Input: part model. Units: mm. Frame: model coordinates. Face numbers are marked on the shaded views. A direction names the side the tool comes from. Give positions to 0.01 mm unless a question says otherwise; leave off trailing zeros. Loops run counter-clockwise (first coordinate to the right, second up) from the corner with the lowest first, then second, coordinate; pieces in that order, holes last.
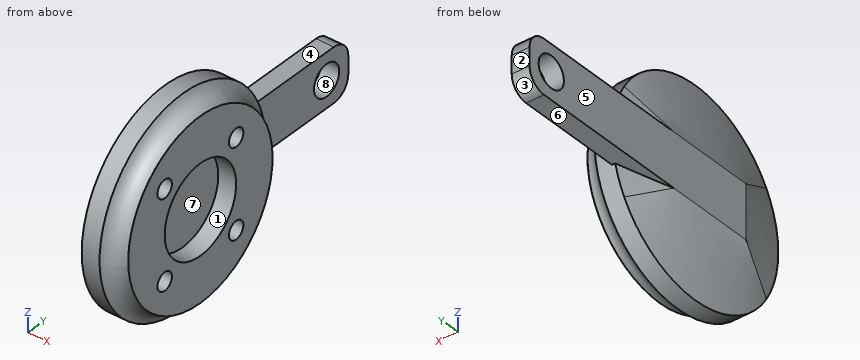
from build123d import *

# Parameters (mm, degrees)
SKETCH1_R           = 11.5
SKETCH1_R_2         = 10.5
BOSS_EXTRUDE1_DEPTH = 2
SKETCH1_2_R         = 10.5
BOSS_EXTRUDE2_DEPTH = 2
SKETCH3_R           = 9.5
CUT_EXTRUDE2_DEPTH  = 1.5
SKETCH6_W           = 30
SKETCH6_H           = 6
SKETCH6_R           = 1.75
BOSS_EXTRUDE3_DEPTH = 2
SKETCH7_R           = 10
SKETCH7_R_2         = 1
SKETCH7_R_3         = 4.95
BOSS_EXTRUDE4_DEPTH = 2
FILLET1_R           = 2
FILLET2_R           = 2


with BuildPart() as part:
    # Sketch1 → Boss-Extrude1 (new body)
    with BuildSketch(Plane.YZ):
        with Locations(Location((0, 0, 0), (0, 0, 270))):
            Circle(SKETCH1_R)
        with Locations(Location((0, 0, 0), (0, 0, 270))):
            Circle(SKETCH1_R_2, mode=Mode.SUBTRACT)
    extrude(amount=BOSS_EXTRUDE1_DEPTH)

    # Sketch1<2> → Boss-Extrude2 (add)
    with BuildSketch(Plane.YZ):
        Circle(SKETCH1_2_R)
    extrude(amount=BOSS_EXTRUDE2_DEPTH)

    # Sketch3 → Cut-Extrude2 (cut)
    with BuildSketch(Plane(origin=(0, 0, 0), x_dir=(0, -1, 0), z_dir=(-1, 0, 0))):
        with Locations(Location((0, 0, 0), (0, 0, 90))):
            Circle(SKETCH3_R)
    extrude(amount=-CUT_EXTRUDE2_DEPTH, mode=Mode.SUBTRACT)

    # Sketch4 for Loft1 → Loft1 section 0
    with BuildSketch(Plane(origin=(0, 0, 0), x_dir=(0, -1, 0), z_dir=(-1, 0, 0))):
        with BuildLine():
            # circular arc as an exact rational Bezier (weights 1, cos(half-angle), 1)
            Bezier((9.861168646, -5.916701187), (13.411189358, 0), (9.861168646, 5.916701187), weights=[1, 0.857492926, 1])
            Bezier((9.861168646, 5.916701187), (0, 22.351982265), (-9.861168646, 5.916701187), weights=[1, 0.514495755, 1])
            Bezier((-9.861168646, 5.916701187), (-13.411189358, 0), (-9.861168646, -5.916701187), weights=[1, 0.857492926, 1])
            Bezier((-9.861168646, -5.916701187), (0, -22.351982265), (9.861168646, -5.916701187), weights=[1, 0.514495755, 1])
        make_face()
    # Sketch2 → Loft1 section 1
    with BuildSketch(Plane.ZY.offset(1.64)):
        with BuildLine():
            Line((-3, -5), (3, -5))
            Line((3, -5), (3, 5))
            Line((3, 5), (-3, 5))
            Line((-3, 5), (-3, -5))
        make_face()
    loft()

    # Sketch6 → Boss-Extrude3 (add)
    with BuildSketch(Plane(origin=(-1.64, 0, 0), x_dir=(0, -1, 0), z_dir=(-1, 0, 0))):
        with Locations((-10, 0)):
            Rectangle(SKETCH6_W, SKETCH6_H)
        with Locations(Location((-22, 0, 0), (0, 0, 90))):
            Circle(SKETCH6_R, mode=Mode.SUBTRACT)
    extrude(amount=-BOSS_EXTRUDE3_DEPTH)

    # Sketch7 → Boss-Extrude4 (add)
    with BuildSketch(Plane.YZ.offset(2)):
        with Locations(Location((0, 0, 0), (0, 0, 270))):
            Circle(SKETCH7_R)
        with Locations(Location((-4.95, 4.95, 0), (0, 0, 270))):
            Circle(SKETCH7_R_2, mode=Mode.SUBTRACT)
        with Locations(Location((4.95, 4.95, 0), (0, 0, 270))):
            Circle(SKETCH7_R_2, mode=Mode.SUBTRACT)
        with Locations(Location((4.95, -4.95, 0), (0, 0, 270))):
            Circle(SKETCH7_R_2, mode=Mode.SUBTRACT)
        with Locations(Location((-4.95, -4.95, 0), (0, 0, 270))):
            Circle(SKETCH7_R_2, mode=Mode.SUBTRACT)
        with Locations(Location((0, 0, 0), (0, 0, 270))):
            Circle(SKETCH7_R_3, mode=Mode.SUBTRACT)
    extrude(amount=BOSS_EXTRUDE4_DEPTH)

    # Fillet1
    # the kernel refuses this fillet: 2 mm, written as the material it adds along each edge
    with BuildSketch(Plane(origin=(2, 0, 0), x_dir=(0, 0, -1), z_dir=(0, -1, 0))) as fillet1_piece_1:
        with BuildLine():
            CenterArc((12, 1.936491673), FILLET1_R, 180, 75.522487814)
            Line((10, 1.936491673), (9.96, 1.936491673))
            Line((9.96, 1.936491673), (9.96, 0))
            Line((9.96, 0), (10, -0.04))
            ThreePointArc((10, -0.04), (10.75, -0.04), (11.49, -0.038729833))
            Line((11.49, -0.038729833), (11.5, 0))
        make_face()
    revolve(axis=Axis((2, 0, 0), (1, 0, 0)))

    # Fillet2
    fillet2_edges = [part.edges().sort_by_distance(p)[0] for p in [
        (-0.64, 25, 3),
        (-0.64, 25, -3),
    ]]
    fillet(fillet2_edges, radius=FILLET2_R)


solid = part.part
(1) Mould query, pull axis Z, two halves, no side actions, for the marked faces 1, 2 and 3. Classes: +Z half, -Z half, draft (parallel to the pull), parting line (faces both ways), or undercut.
Values follow:
face 1: undercut
face 2: draft
face 3: -Z half
(2) Ray query, probe 1 along Y at (x, z) = (3.5, 4.25); probe 2 along X at (y, z) = (-1, -6.25); probe 3 along Z at (x, y) = (-1, 12.5). Return the intervals inside material, ascending.
Values follow:
probe 1: y = -9.11 to -5.66, -4.24 to -2.54, 2.54 to 4.24, 5.66 to 9.11
probe 2: x = -1 to 0, 1.5 to 4
probe 3: z = -3 to 3
(3) Pin query (flat end, axial travel): pin 1 Ø1 at (x, y) = (0, 14.5) entering from +Z; pin 2 Ø2.5 at (y, z) = (-4.95, 4.95) entering from -X; pin 3 Ø1.8 at (y, z) = (4.95, -4.95) entering from -X. Return the tip coordinate at first contact, or that it passes through.
Values follow:
pin 1: stops at z = 3
pin 2: stops at x = -1.38
pin 3: stops at x = -1.29
(4) Cut plane B-B (x = 3.1). Return the cut outline in (y, z).
Values follow:
outline: circle Ø20.37 at (0, 0); hole circle Ø2 at (-4.95, -4.95); hole circle Ø2 at (-4.95, 4.95); hole circle Ø9.9 at (0, 0); hole circle Ø2 at (4.95, -4.95); hole circle Ø2 at (4.95, 4.95)
(5) Reachability of the marked faces 4, 5, 6, 7 and 8 from +Z, -Z, +X, -X, +Y, -Y: full face, straight path, thin tool, end or side. Return the list, or none.
Values follow:
face 4: +Z, -X, +Y
face 5: +Z, -Z, -X, +Y, -Y
face 6: -Z, -X, +Y
face 7: +X
face 8: +X, -X
(6) Cut plane C-C (y = 12). Return the cut outline in (x, z).
Values follow:
outline: (-1.64, -3) - (0.36, -3) - (0.36, 3) - (-1.64, 3) - close
(7) Cut plane A-A (y = 22). Return the cut outline in (x, z), and give its area (3 significant figures).
Values follow:
outline: (-1.64, -3) - (0.36, -3) - (0.36, -1.75) - (-1.64, -1.75) - close; (-1.64, 1.75) - (0.36, 1.75) - (0.36, 3) - (-1.64, 3) - close
area: 5.00 mm2
